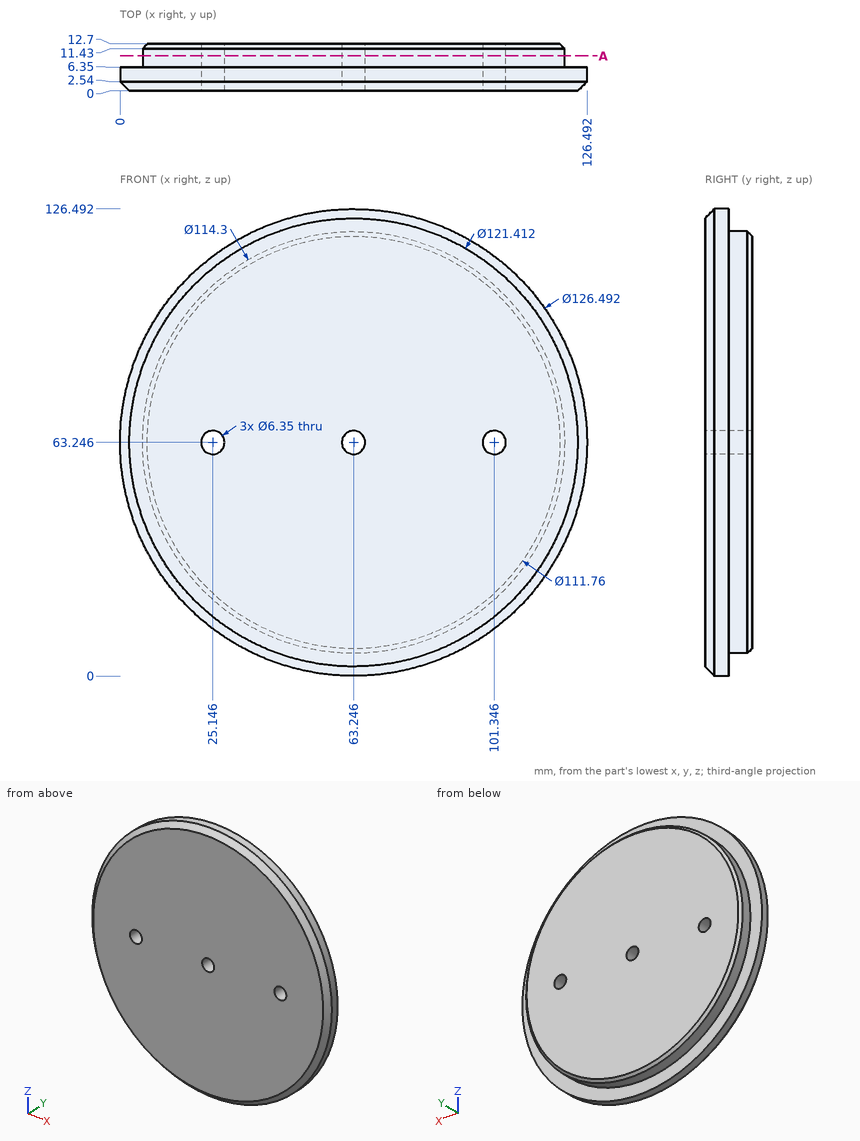
Part print with two shaded views. Sizes in mm from the minimum x, y, z corner. Round coordinates to 2 decimals unless told otherwise and drop trailing zeros. Loops run counter-clockwise (first coordinate to the right, second up) from the corner with the lowest first, then second, coordinate; pieces in that order, holes last. Notation, with made-up numbers: (68, 47.25) - (107, 47.25) arc R21 ccw to (107, 75.25) - close; hole circle Ø11 at (-12.75, -9.5). An arc over 180 degrees is marked (long way). Put each result on its own line as item: value.
1. Pin check, flat tips, straight feed: P1, Ø1.5, axis at x = 23, y = 2.5, coming from the +Z side; P2, Ø5, axis at y = 10.5, z = 79, coming from the +X side; P3, Ø5, axis at y = 4.5, z = 92.5, coming from the +X side. Stop position of each tip, or through.
Geometry check:
P1: z = 112.64
P2: x = 118.84
P3: x = 120.55
2. Slice it at A-A on y = 9.5. List the corners of the cut face in (x, z) (3 decimals), and give its area (3 significant figures).
Geometry check:
outline: circle Ø114.3 at (63.246, 63.246); hole circle Ø6.35 at (25.146, 63.246); hole circle Ø6.35 at (63.246, 63.246); hole circle Ø6.35 at (101.346, 63.246)
area: 10,200 mm²
3. Wall check: line 1 (Z direction, x = 63, y = 4); line 2 (Y direction, x = 26, z = 15.5); line 3 (Z direction, x = 28.5, y = 7). Give the ranges that are in metal, low to high.
Geometry check:
line 1: 0 to 60.08, 66.41 to 126.49
line 2: 0 to 6.35
line 3: 17.87 to 108.62
